Answer from the drawing. Dimensions are ordinates in mm from the lowest x, y and z of the part. Coordinates: 2 decimals unless noted, no trailing zeros. Write each loop counter-clockwise with the first axis right and the second up, starting at its lowest first coordinate (ties: lowest second). Pieces come first, ordered by that corner, then holes. Notation, with made-up numbers: (51.25, 68.25) -> (69.25, 68.25) arc R15 ccw to (69.25, 95.25) -> close; hole circle Ø6 at (39, 70.25). An arc over 180 degrees is marked (long way). One line per item, written item: value. Start each with the question number.
1. Find section D-D, the plane y = 35. Write down the section's boundary in (x, z), and give its area (3 significant figures).
2. Consider line 1 along Y through (x, z) = (3.9, 4.5); line 2 along Y through (x, z) = (1.85, 55); line 3 along Z through (x, y) = (2.4, 16.5) (1 decimal). Determine where each line is inside the solid, lowest interval first.
3. Given P1, Ø10.5, axis at y = 20, z = 55, coming from the +X side; P2, Ø2.5, axis at x = 3.5, y = 70.5, coming from the -Z side; P3, Ø6.5, axis at y = 59.76, z = 65, coming from the -X side; P4, Ø3, axis at x = 2, y = 29.5, coming from the +Z side, each flat-ended and moving along its own axis, determine where each tip first touches the part or whether it passes through.
4. Find section A-A, the plane z = 55. Write down the section's boundary in (x, y).
5. Find section B-B, the plane x = 0.8. Write down the section's boundary in (y, z) (1 decimal), and give its area (3 significant figures).
6. Find section C-C, the plane z = 65. Write down the section's boundary in (x, y), and give its area (3 significant figures).
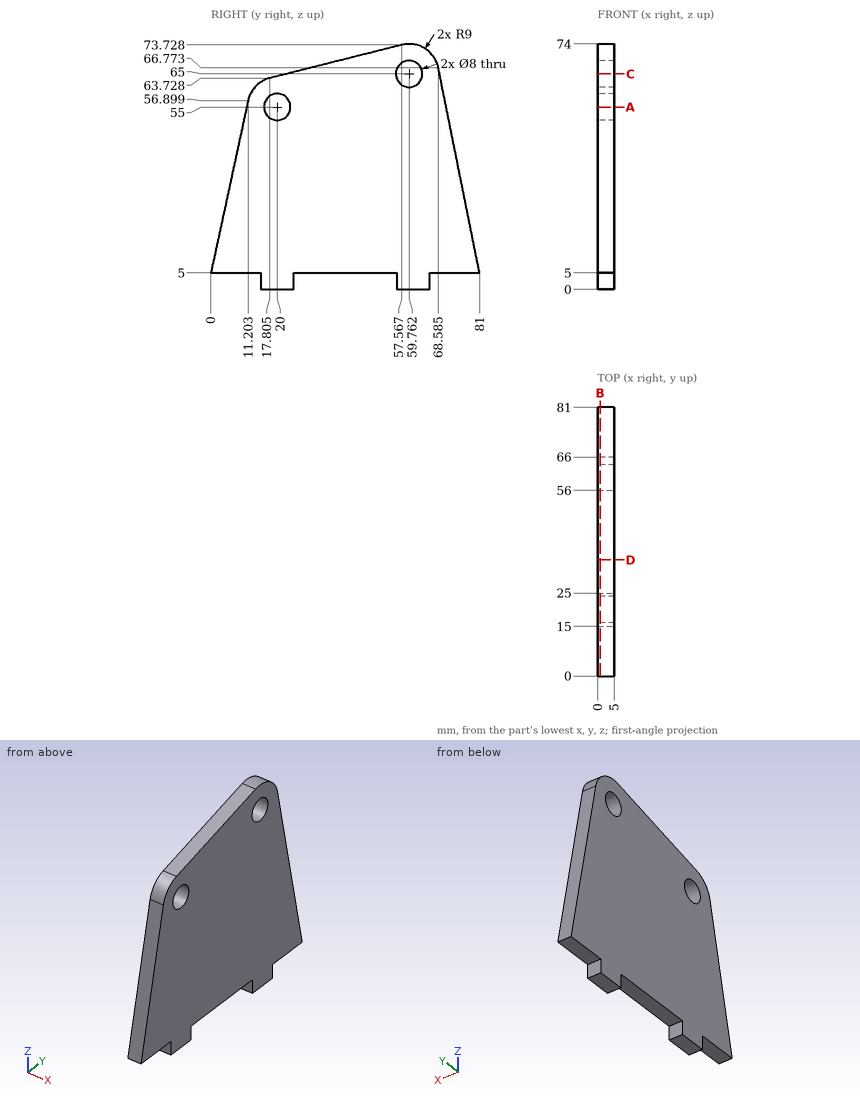
Answer block:
1. outline: (0, 5) -> (5, 5) -> (5, 68.05) -> (0, 68.05) -> close
1. area: 315 mm2
2. line 1: y = 15 to 25, 56 to 66
2. line 2: y = 10.79 to 16, 24 to 70.95
2. line 3: z = 0 to 53.1, 56.9 to 63.3
3. P1: stops at x = 5
3. P2: stops at z = 5
3. P3: passes through
3. P4: stops at z = 67.05
4. outline: (0, 10.79) -> (5, 10.79) -> (5, 16) -> (0, 16) -> close; (0, 24) -> (5, 24) -> (5, 70.95) -> (0, 70.95) -> close
5. outline: (0, 5) -> (15, 5) -> (15, 0) -> (25, 0) -> (25, 5) -> (56, 5) -> (56, 0) -> (66, 0) -> (66, 5) -> (81, 5) -> (68.6, 66.8) arc R9 ccw to (57.6, 73.7) -> (17.8, 63.7) arc R9 ccw to (11.2, 56.9) -> close; hole circle Ø8 at (20, 55); hole circle Ø8 at (59.8, 65)
5. area: 4,330 mm2
6. outline: (0, 22.86) -> (5, 22.86) -> (5, 55.76) -> (0, 55.76) -> close; (0, 63.76) -> (5, 63.76) -> (5, 68.94) -> (0, 68.94) -> close
6. area: 190 mm2
